Here's how the part is built. I have some questions about the finished solid (model axes, mm). Face numbers are marked on the shaded views. A direction names the side the tool comes from. Give positions to 0.01 mm unless a question says otherwise; leave off trailing zeros. Loops run counter-clockwise (first coordinate to the right, second up) from the corner with the lowest first, then second, coordinate; pieces in that order, holes last. Notation, with made-up numbers: (-34, 36.5) - (-26, 36.5) arc R20 cw to (-26, 56.5) - close; hole circle Ø1 at (-27, -7.5). An arc over 180 degrees is marked (long way). One line per item, written item: value. Start each with the question number.
```python
from build123d import *

# Parameters (mm, degrees)
SKETCH_1_W               = 132
SKETCH_1_H               = 42
EXTRUDE_1_DEPTH          = 4
SKETCH_2_R               = 2
SKETCH_2_R_2             = 13.5
CUT_EXTRUDE_1_DEPTH      = 4
SKETCH_3_W               = 4
SKETCH_3_H               = 42
EXTRUDE_2_DEPTH          = 30
SKETCH_4_W               = 58
SKETCH_4_H               = 42
EXTRUDE_3_DEPTH          = 4
SKETCH_5_W               = 4
SKETCH_5_H               = 42
EXTRUDE_4_DEPTH          = 20
SKETCH_6_R               = 7.5
SKETCH_6_R_2             = 2.5
CUT_EXTRUDE_2_DEPTH      = 4
CUT_EXTRUDE_3_DEPTH      = 105.450945424
FILLET_1_R               = 3
SKETCH_8_W               = 37
SKETCH_8_H               = 6.5
CUT_EXTRUDE_4_DEPTH      = 24
FILLET_2_R               = 20
CUT_EXTRUDE_6_DEPTH      = 105.450945424
CUT_EXTRUDE_7_DEPTH      = 139.956827828
CUT_EXTRUDE_7_DEPTH_BACK = 139.956827828
SKETCH_12_R              = 1.5
FILLET_5_R               = 3
FILLET_6_R               = 5


with BuildPart() as part:
    # 草图1 → 凸台-拉伸1 (new body)
    with BuildSketch(Plane(origin=(0, 0, 0), x_dir=(1, 0, 0), z_dir=(0, 1, 0))):
        Rectangle(SKETCH_1_W, SKETCH_1_H)
    extrude(amount=EXTRUDE_1_DEPTH)

    # 草图2 → 切除-拉伸1 (cut)
    with BuildSketch(Plane(origin=(0, 4, 0), x_dir=(1, 0, 0), z_dir=(0, 1, 0))):
        with Locations(Location((12.374368671, 12.374368671, 0), (0, 0, 270))):
            Circle(SKETCH_2_R)
        with Locations(Location((12.374368671, -12.374368671, 0), (0, 0, 270))):
            Circle(SKETCH_2_R)
        with Locations(Location((-12.374368671, -12.374368671, 0), (0, 0, 270))):
            Circle(SKETCH_2_R)
        with Locations(Location((-12.374368671, 12.374368671, 0), (0, 0, 270))):
            Circle(SKETCH_2_R)
        with Locations(Location((0, 0, 0), (0, 0, 270))):
            Circle(SKETCH_2_R_2)
    extrude(amount=-CUT_EXTRUDE_1_DEPTH, mode=Mode.SUBTRACT)

    # 草图3 → 凸台-拉伸2 (add)
    with BuildSketch(Plane(origin=(0, 4, 0), x_dir=(1, 0, 0), z_dir=(0, 1, 0))):
        with Locations((27, 0)):
            Rectangle(SKETCH_3_W, SKETCH_3_H)
        with Locations((-27, 0)):
            Rectangle(SKETCH_3_W, SKETCH_3_H)
    extrude(amount=EXTRUDE_2_DEPTH)

    # 草图4 → 凸台-拉伸3 (add)
    with BuildSketch(Plane(origin=(0, 34, 0), x_dir=(1, 0, 0), z_dir=(0, 1, 0))):
        Rectangle(SKETCH_4_W, SKETCH_4_H)
    extrude(amount=EXTRUDE_3_DEPTH)

    # 草图5 → 凸台-拉伸4 (add)
    with BuildSketch(Plane.XZ):
        with Locations((64, 0)):
            Rectangle(SKETCH_5_W, SKETCH_5_H)
        with Locations((-64, 0)):
            Rectangle(SKETCH_5_W, SKETCH_5_H)
    extrude(amount=EXTRUDE_4_DEPTH)

    # 草图6 → 切除-拉伸2 (cut)
    with BuildSketch(Plane(origin=(0, 38, 0), x_dir=(1, 0, 0), z_dir=(0, 1, 0))):
        with Locations(Location((0, 0, 0), (0, 0, 270))):
            Circle(SKETCH_6_R)
        with Locations(Location((-18.5, 0, 0), (0, 0, 270))):
            Circle(SKETCH_6_R_2)
        with Locations(Location((18.5, 0, 0), (0, 0, 90))):
            Circle(SKETCH_6_R_2)
    extrude(amount=-CUT_EXTRUDE_2_DEPTH, mode=Mode.SUBTRACT)

    # 草图7 → 切除-拉伸3 (cut, through all)
    with BuildSketch(Plane.ZY.offset(29)):
        Polygon((-21, 4), (-12.5, 34), (-12.5, 38), (-21, 38), align=None)
        Polygon((21, 38), (12.5, 38), (12.5, 34), (21, 4), align=None)
    extrude(amount=-CUT_EXTRUDE_3_DEPTH, mode=Mode.SUBTRACT)

    # 圆角1
    fillet_1_edges = [part.edges().sort_by_distance(p)[0] for p in [
        (-27, 34, -12.5),
        (27, 34, -12.5),
        (27, 34, 12.5),
        (-27, 34, 12.5),
    ]]
    fillet(fillet_1_edges, radius=FILLET_1_R)

    # 草图8 → 切除-拉伸4 (cut)
    with BuildSketch(Plane(origin=(0, 4, 0), x_dir=(1, 0, 0), z_dir=(0, 1, 0))):
        Polygon((-66, 5.5), (-66, 21), (-29, 21), (-29, 5.5), (-62, 5.5), align=None)
        with Locations((47.5, -17.75)):
            Rectangle(SKETCH_8_W, SKETCH_8_H)
        Polygon((66, 5.5), (66, 21), (29, 21), (29, 5.5), (62, 5.5), align=None)
        with Locations((-47.5, -17.75)):
            Rectangle(SKETCH_8_W, SKETCH_8_H)
    extrude(amount=-CUT_EXTRUDE_4_DEPTH, mode=Mode.SUBTRACT)

    # 圆角2
    # the kernel refuses this fillet: 20 mm, written as the material it adds along each edge
    with BuildSketch(Plane(origin=(29, 4, 14.5), x_dir=(0, 0, 1), z_dir=(0, -1, 0))) as fillet_2_piece_1:
        with BuildLine():
            CenterArc((20, -14.756354563), FILLET_2_R, 132.454150204, 47.545849796)
            Line((0, -14.756354563), (0, 0))
            Line((0, 0), (6.5, 0))
        make_face()
    extrude(amount=4)
    with BuildSketch(Plane(origin=(29, 4, -5.5), x_dir=(0, 0, -1), z_dir=(0, -1, 0))) as fillet_2_piece_2:
        with BuildLine():
            CenterArc((20, 19.48717527), FILLET_2_R, 180, 76.997121837)
            Line((0, 19.48717527), (0, 0))
            Line((0, 0), (15.5, 0))
        make_face()
    extrude(amount=4)
    with BuildSketch(Plane(origin=(-29, 4, -5.5), x_dir=(0, 0, -1), z_dir=(0, -1, 0))) as fillet_2_piece_3:
        with BuildLine():
            CenterArc((20, -19.48717527), FILLET_2_R, 103.002878163, 76.997121837)
            Line((0, -19.48717527), (0, 0))
            Line((0, 0), (15.5, 0))
        make_face()
    extrude(amount=4)
    with BuildSketch(Plane(origin=(-29, 4, 14.5), x_dir=(0, 0, 1), z_dir=(0, -1, 0))) as fillet_2_piece_4:
        with BuildLine():
            CenterArc((20, 14.756354563), FILLET_2_R, 180, 47.545849796)
            Line((0, 14.756354563), (0, 0))
            Line((0, 0), (6.5, 0))
        make_face()
    extrude(amount=4)

    # 草图11 → 切除-拉伸6 (cut, through all)
    with BuildSketch(Plane.ZY.offset(29)):
        Polygon((8.719846057, 29), (-8.719846057, 29), (-14.386512724, 9), (14.386512724, 9), align=None)
    extrude(amount=-CUT_EXTRUDE_6_DEPTH, mode=Mode.SUBTRACT)

    # 草图12 → 切除-拉伸7 (cut, two sides: drawn at the far end of the back side and taken through both)
    with BuildSketch(Plane.ZY.offset(66).offset(-CUT_EXTRUDE_7_DEPTH_BACK)):
        with Locations((-1.5, -4)):
            Circle(SKETCH_12_R)
        with Locations(Location((10.5, -4, 0), (0, 0, 180))):
            Circle(SKETCH_12_R)
        with Locations((10.5, -16)):
            Circle(SKETCH_12_R)
        with Locations(Location((-1.5, -16, 0), (0, 0, 180))):
            Circle(SKETCH_12_R)
    extrude(amount=CUT_EXTRUDE_7_DEPTH + CUT_EXTRUDE_7_DEPTH_BACK, mode=Mode.SUBTRACT)

    # 圆角5
    fillet_5_edges = [part.edges().sort_by_distance(p)[0] for p in [
        (64, -20, -5.5),
        (-64, -20, 14.5),
        (64, -20, 14.5),
        (-64, -20, -5.5),
    ]]
    fillet(fillet_5_edges, radius=FILLET_5_R)

    # 圆角6
    fillet_6_edges = [part.edges().sort_by_distance(p)[0] for p in [
        (-27, 29, 8.719846057),
        (27, 29, 8.719846057),
        (-27, 9, 14.386512724),
        (27, 9, 14.386512724),
        (-27, 9, -14.386512724),
        (27, 9, -14.386512724),
        (-27, 29, -8.719846057),
        (27, 29, -8.719846057),
    ]]
    fillet(fillet_6_edges, radius=FILLET_6_R)


solid = part.part
```
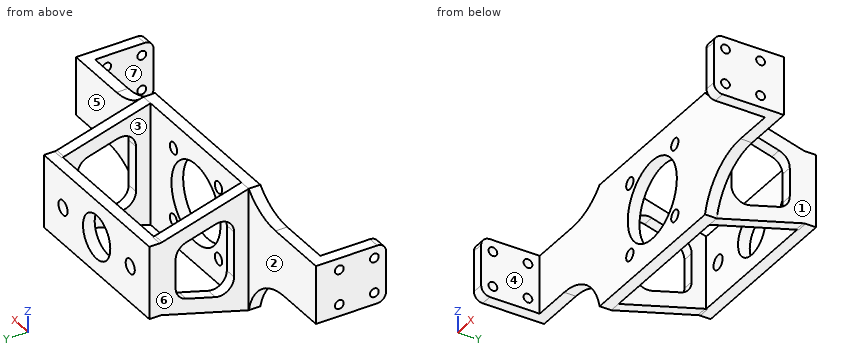
(1) If we section it at B-B on y = -4: List the corners of the cut face in (x, z) for me.
(2) Please list where these lines run through material, in increasing order: probe 1 along X at (y, z) = (35.25, 0); probe 2 along Y at (x, z) = (-62.85, -1.5); probe 3 along X at (y, z) = (-15.5, 9). Write a range as from..to.
(3) If we section it at A-A on x = 23: List the corners of the cut face in (y, z) for me.
(4) If we section it at C-C on x = 0: List the corners of the cut face in (y, z) for me, plus the area to 3 significant figures.
(5) If we section it at D-D on y = 5.5: List the corners of the cut face in (x, z) for me (3 decimals), plus the area to 3 significant figures.
(6) Will these pins go through, and if not, where does the flat tip stop? pin 1 (1 mm diameter, centred on y = 24, z = -11, fed in from +X); pin 2 (23 mm diameter, centred on x = 52.5, y = -4.5, fed in from +Z); pin 3 (5 mm diameter, centred on x = -12.37, z = -12.37, fed in from -Y).
(7) For the marked faces 1, 2, 3 and 4, which set-ups out of +Z, -Z, +X, -X, +Y, -Y let a thin tool reach every point of the face, with its end or its side?
(8) If we mould it in two halves opening along X, with no side actions, what happens to the marked faces 5, 6 and 7? For each: pulls with the +X half, pulls with the -X half, needs draft (parallel to the pull), parting line crosses it, or undercut.
Found:
1. outline: (-66, -5.5) - (-62, -5.5) - (-62, -3) - (-66, -3) - close; (-66, 0) - (-62, 0) - (-62, 9) - (-66, 9) - close; (-66, 12) - (-62, 12) - (-62, 14.5) - (-66, 14.5) - close; (62, -5.5) - (66, -5.5) - (66, -3) - (62, -3) - close; (62, 0) - (66, 0) - (66, 9) - (62, 9) - close; (62, 12) - (66, 12) - (66, 14.5) - (62, 14.5) - close
2. probe 1: -29..-21, -16..-7.5, 7.5..16, 21..29
2. probe 2: -20..-17.5, -14.5..-5.5, -2.5..4
2. probe 3: -66..-62, 62..66
3. outline: (0, -21) - (4, -21) - (4, 21) - (0, 21) - close; (34, -12.5) - (38, -12.5) - (38, 12.5) - (34, 12.5) - close
4. outline: (0, -21) - (4, -21) - (4, -13.5) - (0, -13.5) - close; (0, 13.5) - (4, 13.5) - (4, 21) - (0, 21) - close; (34, -12.5) - (38, -12.5) - (38, -7.5) - (34, -7.5) - close; (34, 7.5) - (38, 7.5) - (38, 12.5) - (34, 12.5) - close
4. area: 100 mm^2
5. outline: (-29, -20.575) - (-25, -20.575) - (-25, 20.575) - (-29, 20.575) - close; (25, -20.575) - (29, -20.575) - (29, 20.575) - (25, 20.575) - close
5. area: 329 mm^2
6. pin 1: x = 29
6. pin 2: z = 14.58
6. pin 3: y = 0
7. face 1: +Z, -Z, +X, +Y
7. face 2: +Z, -Z, -X, +Y
7. face 3: +Z, -Z
7. face 4: +Z, -Z, -Y
8. face 5: needs draft
8. face 6: pulls with the -X half
8. face 7: undercut
